Verification items for the finished model (mm, model axes). A direction names the side the tool comes from. Give positions to 0.01 mm unless a question says otherwise; leave off trailing zeros. Loops run counter-clockwise (first coordinate to the right, second up) from the corner with the lowest first, then second, coordinate; pieces in that order, holes last. Notation, with made-up numbers: (75, -11) -> (81, -11) arc R24 cw to (81, 16) -> close; hole circle Ø11 at (82, 3). An arc over 180 degrees is marked (long way). Answer in a Markdown table with one row per item. Add a question column.
Q1. Release check for a two-part mould opening along X. For faces 3 (the face through (0, -33.02, 61)), 4 (the face through (-1.439, 27.385, 130.666)), 5 (the face through (27.56, 27, 61)) record: pulls with the +X half, pulls with the -X half, needs draft (parallel to the pull), parting line crosses it, or undercut.
Q2. Material ranges on probe 1 along Z at (x, y) = (0, 26); probe 2 along Y at (x, z) = (18, 108.5); probe 3 along Z at (x, y) = (2, 25.5), recorded low to high.
Q3. Set-up check for faces 1 (the face through (12.72, -0.46, -24.45)), 2 (the face through (0, 33.02, 61)): record each of +Z, -Z, +X, -X, +Y, -Y from which the full face is reachable in a straight line by a thin tool's end or side.
Q4. Section check A-A on x = 0. Enter the section's corners in (y, z), and give its area (3 significant figures).
Q5. Section check C-C on y = -11.5. Enter the section's corners in (x, z).
Q6. Section check B-B on z = 41.5. Enter the section's corners in (x, y).
Q7. Section check D-D on x = -14.5. Enter the section's corners in (y, z), and give its area (3 significant figures).
Q8. Gauge pin test, flat ends, axial feed: P1, Ø12, axis at x = 14, y = 22.5, coming from the +Z side; P2, Ø10, axis at x = -13, y = -21, coming from the -Z side; P3, Ø2, axis at x = 20, y = -18, coming from the -Z side; P4, Ø17.5, axis at x = 0, z = 0, coming from the +Y side. Record the tip position at first contact, or that the pin passes through.
```python
from build123d import *

# Parameters (mm, degrees)
F0_R     = 27.560129
F0_R_2   = 11.050129
F1_DEPTH = 33.02
F3_DEPTH = 11.43
F5_DEPTH = 11.43


with BuildPart() as f1:
    # F0 (on Front) → F1 (new body, symmetric)
    with BuildSketch(Plane.XZ):
        Circle(F0_R)
        Circle(F0_R_2, mode=Mode.SUBTRACT)
    extrude(amount=F1_DEPTH, both=True)

    # F2 (on face) → F3 (join)
    with BuildSketch(Plane.XZ.offset(33.02)):
        with BuildLine():
            Line((-27.560129, 119.717821), (-27.560129, 0))
            ThreePointArc((-27.560129, 0), (0, 27.560129), (27.560129, 0))
            Line((27.560129, 0), (27.560129, 119.717821))
            ThreePointArc((27.560129, 119.717821), (0, 92.157692), (-27.560129, 119.717821))
        make_face()
        with BuildLine():
            ThreePointArc((27.560129, 119.717821), (0, 147.277951), (-27.560129, 119.717821))
            Line((-27.560129, 119.717821), (-11.050129, 119.717821))
            ThreePointArc((-11.050129, 119.717821), (0, 130.767951), (11.050129, 119.717821))
            Line((11.050129, 119.717821), (27.560129, 119.717821))
        make_face()
        with BuildLine():
            Line((-11.050129, 119.717821), (-27.560129, 119.717821))
            ThreePointArc((-27.560129, 119.717821), (0, 92.157692), (27.560129, 119.717821))
            Line((27.560129, 119.717821), (11.050129, 119.717821))
            ThreePointArc((11.050129, 119.717821), (0, 108.667692), (-11.050129, 119.717821))
        make_face()
    extrude(amount=-F3_DEPTH)

    # F4 (on face) → F5 (join)
    with BuildSketch(Plane(origin=(0, 33.02, 0), x_dir=(-1, 0, 0), z_dir=(0, 1, 0))):
        with BuildLine():
            Line((-27.560129, 119.7102), (-27.560129, 0))
            ThreePointArc((-27.560129, 0), (0, 27.560129), (27.560129, 0))
            Line((27.560129, 0), (27.560129, 119.7102))
            ThreePointArc((27.560129, 119.7102), (0, 92.150071), (-27.560129, 119.7102))
        make_face()
        with BuildLine():
            Line((-11.050129, 119.7102), (-27.560129, 119.7102))
            ThreePointArc((-27.560129, 119.7102), (0, 92.150071), (27.560129, 119.7102))
            Line((27.560129, 119.7102), (11.050129, 119.7102))
            ThreePointArc((11.050129, 119.7102), (0, 108.660071), (-11.050129, 119.7102))
        make_face()
        with BuildLine():
            ThreePointArc((27.560129, 119.7102), (0, 147.270329), (-27.560129, 119.7102))
            Line((-27.560129, 119.7102), (-11.050129, 119.7102))
            ThreePointArc((-11.050129, 119.7102), (0, 130.760329), (11.050129, 119.7102))
            Line((11.050129, 119.7102), (27.560129, 119.7102))
        make_face()
    extrude(amount=-F5_DEPTH)


solid = f1.part
```
Taken from the geometry:
| question | item | result |
|---|---|---|
| 1 | face 3 | needs draft |
| 1 | face 4 | undercut |
| 1 | face 5 | pulls with the +X half |
| 2 | probe 1 | z = -27.56 to -11.05, 11.05 to 108.66, 130.76 to 147.27 |
| 2 | probe 2 | y = -33.02 to -21.59, 21.59 to 33.02 |
| 2 | probe 3 | z = -27.49 to -10.87, 10.87 to 108.84, 130.58 to 147.2 |
| 3 | face 1 | none |
| 3 | face 2 | +Z, -Z, +X, -X, +Y |
| 4 | outline | (-33.02, -27.56) -> (33.02, -27.56) -> (33.02, -11.05) -> (-33.02, -11.05) -> close; (-33.02, 11.05) -> (33.02, 11.05) -> (33.02, 108.66) -> (21.59, 108.66) -> (21.59, 27.56) -> (-21.59, 27.56) -> (-21.59, 108.67) -> (-33.02, 108.67) -> close; (-33.02, 130.77) -> (-21.59, 130.77) -> (-21.59, 147.28) -> (-33.02, 147.28) -> close; (21.59, 130.76) -> (33.02, 130.76) -> (33.02, 147.27) -> (21.59, 147.27) -> close |
| 4 | area | 4,410 mm² |
| 5 | outline | circle Ø55.12 at (0, 0); hole circle Ø22.1 at (0, 0) |
| 6 | outline | (-27.56, -33.02) -> (27.56, -33.02) -> (27.56, -21.59) -> (-27.56, -21.59) -> close; (-27.56, 21.59) -> (27.56, 21.59) -> (27.56, 33.02) -> (-27.56, 33.02) -> close |
| 7 | outline | (-33.02, -23.44) -> (33.02, -23.44) -> (33.02, 143.15) -> (21.59, 143.15) -> (21.59, 23.44) -> (-21.59, 23.44) -> (-21.59, 143.16) -> (-33.02, 143.16) -> close |
| 7 | area | 5,830 mm² |
| 8 | P1 | stops at z = 146.08 |
| 8 | P2 | stops at z = -26.37 |
| 8 | P3 | stops at z = -19.96 |
| 8 | P4 | passes through |
